Geometry check sheet. Reference: the model listing, model coordinates, mm. Coordinates: 2 decimals unless noted, no trailing zeros. Write each loop counter-clockwise with the first axis right and the second up, starting at its lowest first coordinate (ties: lowest second). Pieces come first, ordered by that corner, then holes. Notation, with made-up numbers: (4.25, -5) -> (27.25, -5) arc R21 ccw to (27.25, 5) -> close; hole circle Ø11 at (18, 57.5). An arc over 180 degrees is marked (long way). One line per question, with ' | ' between items.
Autodesk Inventor part; units mm, degrees
ref_plane "YZ Plane" through (0, 0, 0) normal (1, 0, 0) x (0, 1, 0)
ref_plane "XZ Plane" through (0, 0, 0) normal (0, 1, 0) x (-1, 0, 0)
ref_plane "XY Plane" through (0, 0, 0) normal (0, 0, 1) x (1, 0, 0)
sketch "Sketch1" plane through (0, 0, 0) normal (0, 0, 1) x (1, 0, 0)
  line L0 (0, 0) -> (152.4, 0)
  line L1 (152.4, 0) -> (152.4, -152.4)
  line L2 (152.4, -152.4) -> (0, -152.4)
  line L3 (0, -152.4) -> (0, 0)
  line L4 (0, -152.4) -> (-50.8, -152.4) construction
  line L5 (-50.8, -152.4) -> (-50.8, 25.4) construction
  line L6 (0, 0) -> (0, -152.4)
  line L7 (-47.625, 25.4) -> (152.4, 25.4) construction
  line L8 (152.4, 25.4) -> (152.4, 0) construction
  line L9 (152.4, 0) -> (0, 0)
  line L10 (-47.625, 0) -> (-47.625, 25.4) construction
  line L11 (-50.8, -152.4) -> (-50.8, 25.4) construction
  line L12 (-50.8, 25.4) -> (-47.625, 25.4) construction
  circle A0 centre (60.96, -60.96) radius 54.61 construction
  circle A1 centre (60.96, -60.96) radius 53.34 construction
  circle A2 centre (60.96, -60.96) radius 17.4625
  line L13 (0, 0) -> (-47.625, 0) construction
  line L14 (0, -152.4) -> (-9.525, -152.4)
  line L15 (-9.525, -152.4) -> (-9.525, 3.175)
  line L16 (-3.175, 9.525) -> (152.4, 9.525)
  line L17 (152.4, 0) -> (152.4, 9.525)
  circle A3 centre (60.96, -60.96) radius 47.2059 construction
  line L18 (-4.7625, 9.525) -> (-4.7625, -152.4) construction
  line L19 (-9.525, 4.7625) -> (152.4, 4.7625) construction
  arc A4 (-3.175, 9.525) -> (-9.525, 3.175) centre (-3.175, 3.175) ccw
  circle A5 centre (26.1804, -128.9845) radius 19.25 construction
  circle A6 centre (122.9069, -124.7235) radius 31.75 construction
  circle A7 centre (122.9069, -124.7235) radius 25.4 construction
  circle A8 centre (141.1251, -107.0244) radius 2.4892 construction
  circle A9 centre (104.6888, -142.4226) radius 2.4892 construction
  line L20 (104.6888, -142.4226) -> (141.1251, -107.0244) construction
  circle A10 centre (60.96, -60.96) radius 57.15 construction
  line L21 (60.96, -60.96) -> (122.9069, -124.7235) construction
  circle A11 centre (73.4969, -121.9141) radius 8.89 construction
  circle A12 centre (73.4969, -121.9141) radius 25.4 construction
  circle A13 centre (41.2385, -108.5294) radius 9.525 construction
  circle A14 centre (41.2385, -108.5294) radius 19.05 construction
  circle A15 centre (26.1804, -128.9845) radius 6.35 construction
  point P0 (-9.525, 9.525)
  point P1 (12.7, 4.7625)
  point P2 (-4.7625, -12.7)
  point P3 (76.2, 4.7625)
  point P4 (139.7, 4.7625)
  point P5 (-4.7625, -76.2)
  point P6 (-4.7625, -139.7)
  dimension "d0" = 152.4
  dimension "d8" = 50.8
  dimension "d12" = 3.175
  dimension "d28" = 152.4
  dimension "d29" = 109.22
  dimension "d30" = 106.68
  dimension "d31" = 60.96
  dimension "d32" = 60.96
  dimension "d33" = 34.925
  dimension "d34" = 9.525
  dimension "d35" = 9.525
  dimension "d41" = 94.4118
  dimension "d42" = 25.4
  dimension "d43" = 22.225
  dimension "d44" = 22.225
  dimension "d45" = 6.35
  dimension "d48" = 63.5
  dimension "d55" = 63.5
  dimension "d67" = 38.5
  dimension "d68" = 63.5
  dimension "d69" = 50.8
  dimension "d70" = 4.9784
  dimension "d71" = 114.3
  dimension "d72" = 17.78
  dimension "d73" = 50.8
  dimension "d74" = 19.05
  dimension "d75" = 38.1
  dimension "d76" = 12.7
extrude "Extrusion1" add sketch "Sketch1" along normal blind 4.7625
hole "Hole1" at (12.7, 4.7625, 0) at (-4.7625, -12.7, 0) at (76.2, 4.7625, 0) at (139.7, 4.7625, 0) at (-4.7625, -76.2, 0) at (-4.7625, -139.7, 0) direction (0, 0, 1) diameter 6.35 end through all
properties part number "Module Plate - Bottom"
(1) Depth check by flat-ended pin: P1, Ø8.5, axis at x = -4.76, y = -139.7, coming from the +Z side; P2, Ø5, axis at x = 76.2, y = 4.76, coming from the -Z side. Enter the tip coordinate at first touch or a pass-through.
Answers below:
P1: stops at z = 4.76 | P2: passes through
(2) Cross-section at A-A (y = -60.96). Record the cut outline in (x, z) (1 decimal), plus the area to 3 significant figures.
Answers below:
outline: (-9.5, 0) -> (43.5, 0) -> (43.5, 4.8) -> (-9.5, 4.8) -> close; (78.4, 0) -> (152.4, 0) -> (152.4, 4.8) -> (78.4, 4.8) -> close | area: 605 mm²
(3) Draft check along X on faces 1 (the face through (-9.525, -76, 2)), 2 (the face through (152.4, -70, 2)), 3 (the face through (88, -70, 4.762)), 4 (the face through (48.09, -72.76, 2.35)). Enter one of: pulls with the +X half, pulls with the -X half, needs draft (parallel to the pull), parting line crosses it, or undercut.
Answers below:
face 1: pulls with the -X half | face 2: pulls with the +X half | face 3: needs draft | face 4: undercut
(4) Cross-section at D-D (x = 76.2). Record the cut outline in (y, z) (1 decimal).
Answers below:
outline: (-152.4, 0) -> (-69.5, 0) -> (-69.5, 4.8) -> (-152.4, 4.8) -> close; (-52.4, 0) -> (1.6, 0) -> (1.6, 4.8) -> (-52.4, 4.8) -> close; (7.9, 0) -> (9.5, 0) -> (9.5, 4.8) -> (7.9, 4.8) -> close
(5) Material ranges on line 1 (Y direction, x = 60.96, z = 1.2) (1 decimal); line 2 (Y direction, x = 12.7, z = 3.2) (1 decimal); line 3 (X direction, y = -139.7, z = 1.55) (1 decimal), recorded low to high.
Answers below:
line 1: y = -152.4 to -78.4, -43.5 to 9.5 | line 2: y = -152.4 to 1.6, 7.9 to 9.5 | line 3: x = -9.5 to -7.9, -1.6 to 152.4
(6) Cross-section at C-C (z = 3.6). Count the separate pieces of the cut face and the enclosed holes in it, plus the area to 3 significant figures.
Answers below:
separate pieces: 1 | enclosed holes: 7 | area: 25,100 mm²
(7) Cross-section at B-B (x = 139.7). Record the cut outline in (y, z) (1 decimal), plus the area to 3 significant figures.
Answers below:
outline: (-152.4, 0) -> (1.6, 0) -> (1.6, 4.8) -> (-152.4, 4.8) -> close; (7.9, 0) -> (9.5, 0) -> (9.5, 4.8) -> (7.9, 4.8) -> close | area: 741 mm²
